from build123d import *

# Parameters (mm, degrees)
SKETCH1_R           = 19
BOSS_EXTRUDE1_DEPTH = 12
SKETCH2_R           = 12
BOSS_EXTRUDE2_DEPTH = 80


with BuildPart() as part:
    # Sketch1 → Boss-Extrude1 (new body)
    with BuildSketch(Plane(origin=(0, 0, 0), x_dir=(1, 0, 0), z_dir=(0, 1, 0))):
        Circle(SKETCH1_R)
    extrude(amount=BOSS_EXTRUDE1_DEPTH)

    # Sketch2 → Boss-Extrude2 (add)
    with BuildSketch(Plane.XZ):
        Circle(SKETCH2_R)
    extrude(amount=BOSS_EXTRUDE2_DEPTH)

    # Sketch3 → Cut-Revolve1 (revolve, cut)
    with BuildSketch(Plane(origin=(0, -70, 0), x_dir=(-1, 0, 0), z_dir=(0, -1, 0))):
        Polygon((0, 22), (0, -22), (2, -22), (2.5, 22), align=None)
    revolve(axis=Axis((0, -70, -23.746840194), (0, 0, 1)), mode=Mode.SUBTRACT)


solid = part.part
The model under review builds one solid part; all positions refer to its coordinate system, in mm. A direction names the side the tool comes from. Give positions to 0.01 mm unless a question says otherwise; leave off trailing zeros. Loops run counter-clockwise (first coordinate to the right, second up) from the corner with the lowest first, then second, coordinate; pieces in that order, holes last. Notation, with made-up numbers: (-11.5, 72.25) -> (8.5, 72.25) arc R24 cw to (8.5, 91.25) -> close; hole circle Ø9 at (-9.5, -10). An arc over 180 degrees is marked (long way). Write each question's results on one line, items separated by ' | '.
1) Take a section at B-B, the plane x = 8. Give the boundary of the cut face in (y, z), plus the area to 3 significant figures.
Conclusion:
outline: (-80, -8.94) -> (0, -8.94) -> (0, -17.23) -> (12, -17.23) -> (12, 17.23) -> (0, 17.23) -> (0, 8.94) -> (-80, 8.94) -> close | area: 1,840 mm^2
2) Tool access review of faces 1 (the face through (8.767, 5.916, 16.856)), 2 (the face through (-11.99, -39.44, 0.53)): name each direction out of +Z, -Z, +X, -X, +Y, -Y from which nothing blocks a thin tool from reaching the whole face with its end or side.
Conclusion:
face 1: +Y, -Y | face 2: -Y
3) Insertion check: pin 1 Ø3 at (y, z) = (-18, 15) entering from -X; pin 2 Ø2 at (y, z) = (-9, -0.5) entering from -X; pin 3 Ø12 at (y, z) = (-15, -8) entering from +X; pin 4 Ø8 at (x, y) = (14, -3) entering from -Z. Each pin has a flat end and moves straight along its axis. Give the tip position at first contact, or say it passes through.
Conclusion:
pin 1: passes through | pin 2: stops at x = -12 | pin 3: stops at x = 11.83 | pin 4: stops at z = -15.23
4) Draft analysis for pull direction Y (two halves, no side actions). For faces 3 (the face through (0, -80, 0)), 4 (the face through (-1.21, -71.9, -0.17)), 5 (the face through (0, 12, 0)), state which applies: pulls with the +Y half, pulls with the -Y half, needs draft (parallel to the pull), parting line crosses it, or undercut.
Conclusion:
face 3: pulls with the -Y half | face 4: undercut | face 5: pulls with the +Y half
5) For line 1 along Y through (x, z) = (-2.5, 14.5); line 2 along Z through (x, y) = (0, -43); line 3 along Z through (x, y) = (5, -74.5), list the stretches that pass through material, from the lowest coordinate up. Write a range as from..to.
Conclusion:
line 1: y = 0..12 | line 2: z = -12..12 | line 3: z = -10.91..10.91
6) Take a section at C-C, the plane y = -13. Give the boundary of the cut face in (x, z).
Conclusion:
outline: circle Ø24 at (0, 0)
7) Take a section at A-A, the plane z = 0. Give the boundary of the cut face in (x, y).
Conclusion:
outline: (-19, 0) -> (-12, 0) -> (-12, -80) -> (12, -80) -> (12, 0) -> (19, 0) -> (19, 12) -> (-19, 12) -> close; hole circle Ø4.5 at (0, -70)
8) Take a section at D-D, the plane z = 6. Give the boundary of the cut face in (x, y), plus the area to 3 significant figures.
Conclusion:
outline: (-18.03, 0) -> (-10.39, 0) -> (-10.39, -80) -> (10.39, -80) -> (10.39, 0) -> (18.03, 0) -> (18.03, 12) -> (-18.03, 12) -> close; hole circle Ø4.36 at (0, -70) | area: 2,080 mm^2
